The listing builds one solid part. Answer for the finished solid, in the listing's coordinates (mm). A direction names the side the tool comes from. Give positions to 0.01 mm unless a question says otherwise; leave off trailing zeros. Write each loop counter-clockwise with the first axis right and the second up, starting at its lowest first coordinate (ties: lowest second). Pieces come first, ordered by that corner, then holes.
```python
from build123d import *

# Parameters (mm, degrees)
F1_DEPTH = 47.0916
F0_R     = 10.16
F2_DEPTH = 15.7734
F3_R     = 3.302


with BuildPart() as f1:
    # F0 (on Top) → F1 (new body)
    with BuildSketch(Plane.XY):
        with BuildLine():
            ThreePointArc((5.848104, -28.095686), (22.607385, -18.270235), (29.211287, 0))
            ThreePointArc((29.211287, 0), (22.607385, 18.270235), (5.848103, 28.095686))
            ThreePointArc((5.848103, 28.095686), (-27.938713, 0), (5.848104, -28.095686))
        make_face()
        with BuildLine():
            ThreePointArc((-12.811478, 4.826), (0.636287, 14.2875), (14.084052, 4.826))
            Line((14.084052, 4.826), (19.165587, 4.826))
            Line((19.165587, 4.826), (19.165587, -4.826))
            Line((19.165587, -4.826), (14.084052, -4.826))
            ThreePointArc((14.084052, -4.826), (0.636287, -14.2875), (-12.811478, -4.826))
            Line((-12.811478, -4.826), (-19.165587, -4.826))
            Line((-19.165587, -4.826), (-19.165587, 4.826))
            Line((-19.165587, 4.826), (-12.811478, 4.826))
        make_face(mode=Mode.SUBTRACT)
        with BuildLine():
            ThreePointArc((-12.811478, -4.826), (-13.651213, 0), (-12.811478, 4.826))
            Line((-12.811478, 4.826), (-19.165587, 4.826))
            Line((-19.165587, 4.826), (-19.165587, -4.826))
            Line((-19.165587, -4.826), (-12.811478, -4.826))
        make_face()
    extrude(amount=F1_DEPTH)

    # F0 (on Top) → F2 (join)
    with BuildSketch(Plane.XY):
        with BuildLine():
            ThreePointArc((5.848103, 28.095686), (22.607385, 18.270235), (29.211287, 0))
            ThreePointArc((29.211287, 0), (22.607385, -18.270235), (5.848104, -28.095686))
            Line((5.848104, -28.095686), (54.611287, -19.05))
            ThreePointArc((54.611287, -19.05), (68.081671, -13.470384), (73.661287, 0))
            ThreePointArc((73.661287, 0), (68.081671, 13.470384), (54.611287, 19.05))
            Line((54.611287, 19.05), (5.848103, 28.095686))
        make_face()
        with Locations((54.611287, 0)):
            Circle(F0_R, mode=Mode.SUBTRACT)
    extrude(amount=F2_DEPTH)

    # F3
    f3_edges = [f1.edges().sort_by_distance(p)[0] for p in [
        (-4.57553, 28.095686, 47.0916),
    ]]
    fillet(f3_edges, radius=F3_R)


solid = f1.part
```
Item 1: Which of the six approach directions +Z, -Z, +X, -X, +Y, -Y give full straight-line access (tool end or side, diameter ignored) to faces 1 (the face through (29.888, -23.636, 7.776)), 2 (the face through (19.166, 0, 23))?
Conclusion:
face 1: +Z, -Z, +X, -Y
face 2: +Z, -Z
Item 2: Consider probe 1 along X at (y, z) = (7, 10); probe 2 along X at (y, z) = (-8, 26); probe 3 along Z at (x, y) = (44.5, -2). Determine where each line is inside the solid, lowest interval first.
Conclusion:
probe 1: x = -27.07 to -11.82, 13.09 to 47.25, 61.98 to 72.33
probe 2: x = -26.8 to -11.2, 12.47 to 28.07
probe 3: z = 0 to 15.77
Item 3: A cutting plane is placed at B-B, the plane z = 14. Count the separate pieces of the cut face and the enclosed holes in it, plus the area to 3 significant figures.
Conclusion:
separate pieces: 1
enclosed holes: 2
area: 3,440 mm2
Item 4: A cutting plane is placed at C-C, the plane x = 60. Give the vertices of the cut face in (y, z), plus the area to 3 significant figures.
Conclusion:
outline: (-18.27, 0) - (-8.61, 0) - (-8.61, 15.77) - (-18.27, 15.77) - close; (8.61, 0) - (18.27, 0) - (18.27, 15.77) - (8.61, 15.77) - close
area: 305 mm2
Item 5: A cutting plane is placed at D-D, the plane x = 31. Give the vertices of the cut face in (y, z).
Conclusion:
outline: (-23.43, 0) - (23.43, 0) - (23.43, 15.77) - (-23.43, 15.77) - close
Item 6: Each of these flat-tipped pins is pushed along its axis until it touches: P1, Ø5.5, axis at x = 15.5, z = 26, coming from the +Y side; P2, Ø5, axis at x = 26.5, z = 11, coming from the -Y side; P3, Ø12, axis at x = 54.61, y = 0, coming from the -Z side; P4, Ø1.5, axis at x = 17.5, z = 34, coming from the -Y side. Where does it stop, or does it pass through?
Conclusion:
P1: stops at y = 25.88
P2: stops at y = -24.73
P3: passes through
P4: stops at y = -23.6
